For this review, take the finished solid that the model builds, in its own axes (mm). Face numbers are marked on the shaded views. A direction names the side the tool comes from. Coordinates: 2 decimals unless noted, no trailing zeros. Write each loop counter-clockwise with the first axis right and the second up, starting at its lowest first coordinate (ties: lowest second). Pieces come first, ordered by that corner, then holes.
1) For the marked faces 1 and 2, list the 3-axis set-ups (+Z, -Z, +X, -X, +Y, -Y) from which the entire face can be reached by the end or side of a thin tool; tool diameter is ignored.
2) Mouldability with a two-part tool opening along Y and no side actions: class the marked faces 3, 4 and 5 as pulls with the +Y half, pulls with the -Y half, needs draft (parallel to the pull), parting line crosses it, or undercut.
3) We need section B-B on x = 0. Write out the cut boundary in (y, z), then the cut area to 3 significant figures.
4) We need section D-D on z = -11.5. Write out the cut boundary in (x, y).
5) Insertion check: P1, Ø1, axis at y = 5, z = -3, coming from the -X side; P2, Ø12, axis at x = 1.5, y = -6.5, coming from the +Z side; P3, Ø1, axis at y = 1.5, z = -13.5, coming from the -X side; P4, Ø8, axis at x = -1.5, z = -11.5, coming from the -Y side. Each pin has a flat end and moves straight along its axis. Give the tip position at first contact, or say it passes through.
6) We need section A-A on y = 0. Write out the cut boundary in (x, z), then the cut area to 3 significant figures.
7) We need section C-C on y = -7. Write out the cut boundary in (x, z), then the cut area to 3 significant figures.
8) To check wall thickness, follow line 1 along Y through (x, z) = (0, -15.25); line 2 along Y through (x, z) = (-2, -16.25); line 3 along X through (y, z) = (9, -2.5). State the ranges of each line that lie inside material, in increasing order.
from build123d import *

# Parameters (mm, degrees)
F3_D           = 2.2
F3_CSINK_D     = 4.3
F3_CSINK_ANGLE = 90


with BuildPart() as f1:
    # F0 (on Front) → F1 (revolve)
    with BuildSketch(Plane.XZ):
        Polygon((-9, -1), (-9, 0), (-17, 0), (-17, -3), (-11.5, -3), (-11.5, -20), (-10.5, -20), (-10.5, -1), align=None)
    revolve(axis=Axis((0, 0, -20.998121), (0, 0, -1)))

    # F3 (through all)
    with Locations(Plane.XY):
        with Locations((-14.5, 0), (14.5, 0)):
            CounterSinkHole(F3_D / 2, F3_CSINK_D / 2, counter_sink_angle=F3_CSINK_ANGLE)


solid = f1.part
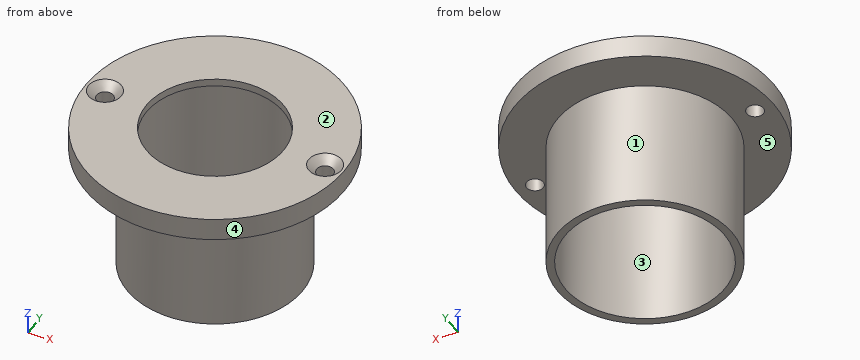
Result:
1. face 1: -Z
1. face 2: +Z, +X, -X, +Y, -Y
2. face 3: undercut
2. face 4: parting line crosses it
2. face 5: needs draft
3. outline: (-17, -3) - (-11.5, -3) - (-11.5, -20) - (-10.5, -20) - (-10.5, -1) - (-9, -1) - (-9, 0) - (-17, 0) - close; (9, -1) - (10.5, -1) - (10.5, -20) - (11.5, -20) - (11.5, -3) - (17, -3) - (17, 0) - (9, 0) - close
3. area: 76.0 mm2
4. outline: circle Ø23 at (0, 0); hole circle Ø21 at (0, 0)
5. P1: stops at x = -16.39
5. P2: stops at z = 0
5. P3: stops at x = -11.46
5. P4: stops at y = -11.5
6. outline: (-17, -3) - (-15.6, -3) - (-15.6, -1.05) - (-16.65, 0) - (-17, 0) - close; (-13.4, -3) - (-11.5, -3) - (-11.5, -20) - (-10.5, -20) - (-10.5, -1) - (-9, -1) - (-9, 0) - (-12.35, 0) - (-13.4, -1.05) - close; (9, -1) - (10.5, -1) - (10.5, -20) - (11.5, -20) - (11.5, -3) - (13.4, -3) - (13.4, -1.05) - (12.35, 0) - (9, 0) - close; (15.6, -3) - (17, -3) - (17, 0) - (16.65, 0) - (15.6, -1.05) - close
6. area: 60.6 mm2
7. outline: (-15.49, -3) - (-9.12, -3) - (-9.12, -20) - (-7.83, -20) - (-7.83, -1) - (-5.66, -1) - (-5.66, 0) - (-15.49, 0) - close; (5.66, -1) - (7.83, -1) - (7.83, -20) - (9.12, -20) - (9.12, -3) - (15.49, -3) - (15.49, 0) - (5.66, 0) - close
7. area: 94.5 mm2
8. line 1: y = -11.5 to -10.5, 10.5 to 11.5
8. line 2: y = -11.32 to -10.31, 10.31 to 11.32
8. line 3: x = -14.42 to -5.41, 5.41 to 14.42
